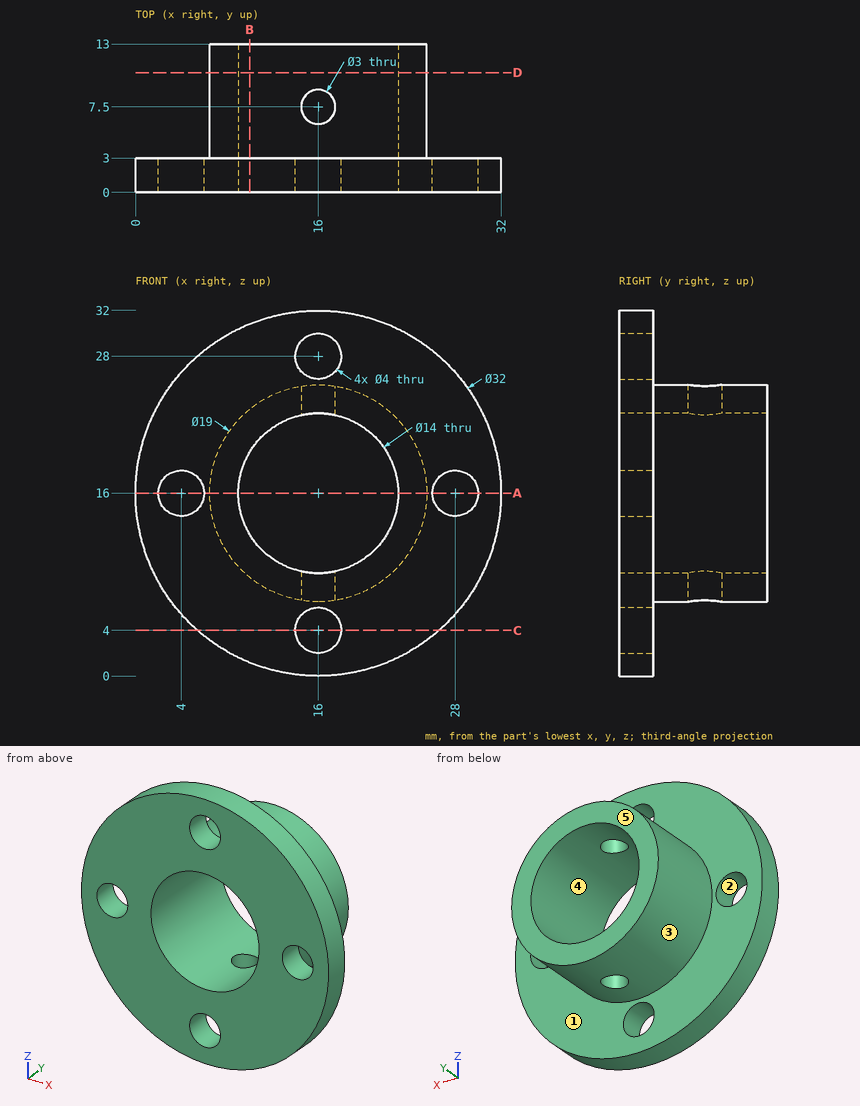
Could you check a few things on this drawing? It's one solid part, dimensions in mm from its lowest x, y, z. A direction names the side the tool comes from. Give positions to 0.01 mm unless a question says otherwise; leave off trailing zeros. Write each loop counter-clockwise with the first axis right and the second up, starting at its lowest first coordinate (ties: lowest second). Pieces come first, ordered by that corner, then holes. Notation, with made-up numbers: (-23.5, 46) -> (7.5, 46) arc R18 ccw to (7.5, 60) -> close; hole circle Ø6 at (24, -29.5). An arc over 180 degrees is marked (long way). Answer as a JSON object with one key per item and string values.
Q1. We'd pull the mould along X, two halves only. Please class the marked faces 3, 4 and 5: released by +X, released by -X, zero draft, split by the parting line, or undercut.
Taken from the geometry:
{"face 3": "split by the parting line", "face 4": "undercut", "face 5": "zero draft"}
Q2. Please list where these lines run through material, in increasing order: L1, parallel to Y at x = 16, z = 7; L2, parallel to X at y = 10.5, z = 16; L3, parallel to Y at x = 27, z = 11.
Taken from the geometry:
{"L1": "y = 0 to 6, 9 to 13", "L2": "x = 6.5 to 9, 23 to 25.5", "L3": "y = 0 to 3"}
Q3. Which directions (+Z, -Z, +X, -X, +Y, -Y) give clear straight access to the entire face, cutting with the end or side of a thin tool? Please do the marked faces 1 and 2.
Taken from the geometry:
{"face 1": "+Y", "face 2": "+Y, -Y"}
Q4. Will these pins go through, and if not, where does the flat tip stop? pin 1 Ø1 at (x, y) = (23, 8) entering from -Z; pin 2 Ø3 at (y, z) = (6.5, 22.5) entering from +X; pin 3 Ø5 at (x, y) = (16, 7.5) entering from -Z.
Taken from the geometry:
{"pin 1": "stops at z = 9.07", "pin 2": "stops at x = 24.08", "pin 3": "stops at z = 6.5"}
Q5. Suppose I cut it at C-C on z = 4. Write out the boundary of the cut face in (x, y).
Taken from the geometry:
{"outline": "(5.42, 0) -> (14, 0) -> (14, 3) -> (5.42, 3) -> close; (18, 0) -> (26.58, 0) -> (26.58, 3) -> (18, 3) -> close"}
Q6. Suppose I cut it at A-A on z = 16. Write out the boundary of the cut face in (x, y), then the cut area to 3 significant figures.
Taken from the geometry:
{"outline": "(0, 0) -> (2, 0) -> (2, 3) -> (0, 3) -> close; (6, 0) -> (9, 0) -> (9, 13) -> (6.5, 13) -> (6.5, 3) -> (6, 3) -> close; (23, 0) -> (26, 0) -> (26, 3) -> (25.5, 3) -> (25.5, 13) -> (23, 13) -> close; (30, 0) -> (32, 0) -> (32, 3) -> (30, 3) -> close", "area": "80.0 mm²"}
Q7. Suppose I cut it at B-B on x = 10. Write out the boundary of the cut face in (y, z).
Taken from the geometry:
{"outline": "(0, 1.17) -> (3, 1.17) -> (3, 8.63) -> (13, 8.63) -> (13, 12.39) -> (0, 12.39) -> close; (0, 19.61) -> (13, 19.61) -> (13, 23.37) -> (3, 23.37) -> (3, 30.83) -> (0, 30.83) -> close"}
Q8. Suppose I cut it at D-D on y = 10.5. Write out the boundary of the cut face in (x, z), then the cut area to 3 significant figures.
Taken from the geometry:
{"outline": "circle Ø19 at (16, 16); hole circle Ø14 at (16, 16)", "area": "130 mm²"}
